```python
from build123d import *

# Parameters (mm, degrees)
EXTRUDE_THIN1_DEPTH = 8
BOSS_EXTRUDE4_DEPTH = 4
SKETCH3_3_R         = 8
CUT_EXTRUDE1_DEPTH  = 4
EXTRUDE_THIN2_DEPTH = 15
FILLET1_R           = 5
FILLET2_R           = 5
SKETCH5_R           = 4
CUT_EXTRUDE2_DEPTH  = 15


with BuildPart() as part:
    # Sketch1 → Extrude-Thin1 (new, symmetric)
    with BuildSketch(Plane.XY):
        with BuildLine():
            Line((0, 0), (-104, 0))
            ThreePointArc((-104, 0), (-115.313708499, 4.686291501), (-120, 16))
            Line((-120, 16), (-120, 60))
            Line((-120, 60), (-116, 60))
            Line((-116, 60), (-116, 16))
            ThreePointArc((-116, 16), (-112.485281374, 7.514718626), (-104, 4))
            Line((-104, 4), (0, 4))
            Line((0, 4), (0, 0))
        make_face()
    extrude(amount=EXTRUDE_THIN1_DEPTH, both=True)

    # Sketch3 → Boss-Extrude4 (add)
    with BuildSketch(Plane(origin=(0, 4, 0), x_dir=(1, 0, 0), z_dir=(0, 1, 0))):
        with BuildLine():
            ThreePointArc((-29.856406461, 8), (-24, 13.856406461), (-16, 16))
            Line((-16, 16), (-56.906606086, 16))
            Line((-56.906606086, 16), (-81.100288315, 8))
            Line((-81.100288315, 8), (-61, 8))
            Line((-61, 8), (-29.856406461, 8))
        make_face()
        with BuildLine():
            ThreePointArc((-2.143593539, 8), (-8, 13.856406461), (-16, 16))
            ThreePointArc((-16, 16), (-24, 13.856406461), (-29.856406461, 8))
            Line((-29.856406461, 8), (-16, 8))
            Line((-16, 8), (-2.143593539, 8))
        make_face()
        with BuildLine():
            Line((-16, -8), (-29.856406461, -8))
            ThreePointArc((-29.856406461, -8), (-24, -13.856406461), (-16, -16))
            ThreePointArc((-16, -16), (-8, -13.856406461), (-2.143593539, -8))
            Line((-2.143593539, -8), (-16, -8))
        make_face()
        with BuildLine():
            ThreePointArc((-16, -16), (-24, -13.856406461), (-29.856406461, -8))
            Line((-29.856406461, -8), (-61, -8))
            Line((-61, -8), (-81.100288315, -8))
            Line((-81.100288315, -8), (-61, -16))
            Line((-61, -16), (-16, -16))
        make_face()
        with BuildLine():
            ThreePointArc((-29.856406461, -8), (-32, 0), (-29.856406461, 8))
            Line((-29.856406461, 8), (-61, 8))
            ThreePointArc((-61, 8), (-55.343145751, 5.656854249), (-53, 0))
            ThreePointArc((-53, 0), (-55.343145751, -5.656854249), (-61, -8))
            Line((-61, -8), (-29.856406461, -8))
        make_face()
    extrude(amount=-BOSS_EXTRUDE4_DEPTH)

    # Sketch3_3 → Cut-Extrude1 (cut)
    with BuildSketch(Plane(origin=(0, 4, 0), x_dir=(1, 0, 0), z_dir=(0, 1, 0))):
        with Locations(Location((-61, 0, 0), (0, 0, 180))):
            Circle(SKETCH3_3_R)
        with Locations(Location((-16, 0, 0), (0, 0, 180))):
            Circle(SKETCH3_3_R)
    extrude(amount=-CUT_EXTRUDE1_DEPTH, mode=Mode.SUBTRACT)

    # Sketch4 → Extrude-Thin2 (add)
    with BuildSketch(Plane(origin=(0, 60, 0), x_dir=(1, 0, 0), z_dir=(0, 1, 0))):
        with BuildLine():
            Line((-120, 8), (-120, 15))
            ThreePointArc((-120, 15), (-119.396926208, 18.420201433), (-117.660444431, 21.427876097))
            Line((-117.660444431, 21.427876097), (-103.519117018, 38.280853845))
            Line((-103.519117018, 38.280853845), (-100.454939246, 35.709703407))
            Line((-100.454939246, 35.709703407), (-114.596266659, 18.856725658))
            ThreePointArc((-114.596266659, 18.856725658), (-115.638155725, 17.05212086), (-116, 15))
            Line((-116, 15), (-116, 8))
            Line((-116, 8), (-120, 8))
        make_face()
    extrude(amount=-EXTRUDE_THIN2_DEPTH)

    # Fillet1
    fillet1_edges = [part.edges().sort_by_distance(p)[0] for p in [
        (-118, 45, -8),
    ]]
    fillet(fillet1_edges, radius=FILLET1_R)

    # Fillet2
    fillet2_edges = [part.edges().sort_by_distance(p)[0] for p in [
        (-101.987028132, 60, -36.995278626),
        (-101.987028132, 45, -36.995278626),
    ]]
    fillet(fillet2_edges, radius=FILLET2_R)

    # Sketch5 → Cut-Extrude2 (cut)
    with BuildSketch(Plane(origin=(-76.532974578, 0, -64.218790741), x_dir=(0.6427876096865437, 0, -0.7660444431189745), z_dir=(0.7660444431189746, 0, 0.6427876096865437))):
        with Locations((-47.215970419, 52.5)):
            Circle(SKETCH5_R)
    extrude(amount=-CUT_EXTRUDE2_DEPTH, mode=Mode.SUBTRACT)


solid = part.part
```
The listing builds one solid part. Answer for the finished solid, in the listing's coordinates (mm). A direction names the side the tool comes from. Coordinates: 2 decimals unless noted, no trailing zeros. Write each loop counter-clockwise with the first axis right and the second up, starting at its lowest first coordinate (ties: lowest second). Pieces come first, ordered by that corner, then holes. Notation, with made-up numbers: M 47.25,24 L 61.25,24 A32 ccw 61.25,63 Z; hole C 65.25,76.5 d7. An arc over 180 degrees is marked long. Use a Markdown table: item, result. Add a question column.
1. Section A-A (z = 0) is taken. Give the vertices of the cut face in (x, y).
2. Straight lines are drawn through the part: line 1 along Z through (x, y) = (-61, 2); line 2 along Z through (x, y) = (-16, 1.8); line 3 along Y through (x, z) = (-44, -11.5). For each, find the intervals that lie inside material, in ascending order. Write a range as [from, to].
3. For a pull along X with two mould halves and no side action, classify faces 1 (the flat face through (-39, 2, 16)), 2 (the flat face through (0, 2, 0)), 3 (the cylindrical face through (-108.951, 48.595, -28.653)), 4 (the cylindrical face through (-54.651, 2.028, -4.868)) as +X half, -X half, draft (parallel to the pull), parting line (faces both ways), or undercut.
4. Section D-D (x = -39) is taken. Give the vertices of the cut face in (y, z), plus the area to 3 significant figures.
5. Section B-B (x = -58.5) is taken. Give the vertices of the cut face in (y, z).
6. Given P1, Ø9.5, axis at x = -16, z = 0, coming from the +Y side; P2, Ø8, axis at x = -68, y = 7, coming from the +Z side; P3, Ø18, axis at x = -114, z = -21.5, coming from the -Y side; P4, Ø6, axis at y = 53.5, z = -13, coming from the +X side, each flat-ended and moving along its own axis, determine where each tip first touches the part or whether it passes through.
7. Which of the six approach directions +Z, -Z, +X, -X, +Y, -Y give full straight-line access (tool end or side, diameter ignored) to faces 5 (the flat face through (-116, 38, -1)), 6 (the cylindrical face through (-112.58, 7.61, 0.11))?
8. Section C-C (y = 47) is taken. Give the vertices of the cut face in (x, z), plus the area to 3 significant figures.
Data:
| question | item | result |
|---|---|---|
| 1 | outline | M -120,16 A16 ccw -104,0 L -69,0 L -69,4 L -104,4 A12 cw -116,16 L -116,60 L -120,60 Z; M -53,0 L -24,0 L -24,4 L -53,4 Z; M -8,0 L 0,0 L 0,4 L -8,4 Z |
| 2 | line 1 | z = [-14.65, -8], [8, 16] |
| 2 | line 2 | z = [-16, -8], [8, 16] |
| 2 | line 3 | y = [0, 4] |
| 3 | face 1 | draft |
| 3 | face 2 | +X half |
| 3 | face 3 | undercut |
| 3 | face 4 | undercut |
| 4 | outline | M 0,-16 L 4,-16 L 4,16 L 0,16 Z |
| 4 | area | 128 mm2 |
| 5 | outline | M 0,-15.47 L 4,-15.47 L 4,-7.6 L 0,-7.6 Z; M 0,7.6 L 4,7.6 L 4,16 L 0,16 Z |
| 6 | P1 | passes through |
| 6 | P2 | stops at z = 14.27 |
| 6 | P3 | stops at y = 44.99 |
| 6 | P4 | stops at x = -115.92 |
| 7 | face 5 | +Z, +X, +Y |
| 7 | face 6 | +Z, -Z, +X, +Y |
| 8 | outline | M -120,-15 A10 ccw -117.66,-21.43 L -104.16,-37.51 L -101.1,-34.94 L -114.6,-18.86 A6 cw -116,-15 L -116,8 L -120,8 Z |
| 8 | area | 198 mm2 |
